```python
from build123d import *

# Parameters (mm, degrees)
F1_DEPTH  = 9.525
F6_DEPTH  = 9.525
F2_R      = 4.7625
F8_DEPTH  = 80.01
F9_W      = 12.7
F9_H      = 19.05
F10_DEPTH = 63.5
F0_W      = 12.7
F0_H      = 12.7
F11_DEPTH = 25.4
F13_DEPTH = 12.7
F14_DEPTH = 9.525


with BuildPart() as f1:
    # F0 (on Top) → F1 (new body, symmetric)
    with BuildSketch(Plane.XY):
        Polygon((-63.5, -44.45), (0, -44.45), (0, -31.75), (-50.8, -31.75), (-50.8, -6.35), (-50.8, 6.35), (-50.8, 31.75), (0, 31.75), (0, 44.45), (-63.5, 44.45), align=None)
    extrude(amount=F1_DEPTH, both=True)

    # F5 (on line) → F6 (cut, symmetric)
    with BuildSketch(Plane(origin=(-20.6375, 0, -20.6375), x_dir=(0, 1, 0), z_dir=(0.7071067812, 0, 0.7071067812))):
        Polygon((-42.8625, 39.9065859181), (-38.1, 37.156955261), (-33.3375, 39.9065859181), (-33.3375, 45.4058472321), (-38.1, 48.1554778891), (-42.8625, 45.4058472321), align=None)
        Polygon((33.3375, 39.9065859181), (38.1, 37.156955261), (42.8625, 39.9065859181), (42.8625, 45.4058472321), (38.1, 48.1554778891), (33.3375, 45.4058472321), align=None)
    extrude(amount=F6_DEPTH, both=True, mode=Mode.SUBTRACT)

    # F7: F1 across plane


with BuildPart() as f1_1:
    add(f1.part)
    add(f1.part.mirror(Plane.YZ))

    # F2 (on Front) → F8 (cut, symmetric)
    with BuildSketch(Plane.XZ):
        Circle(F2_R)
        Polygon((-10.4086411192, -0.79375), (-8.1172822383, 3.175), (-10.4086411192, 7.14375), (-14.9913588808, 7.14375), (-17.2827177617, 3.175), (-14.9913588808, -0.79375), align=None)
    extrude(amount=F8_DEPTH, both=True, mode=Mode.SUBTRACT)

    # F9 (on face) → F10 (join)
    with BuildSketch(Plane.XZ.offset(-31.75)):
        with Locations((-13.97, 0)):
            Rectangle(F9_W, F9_H)
        Polygon((-14.9913588808, -0.79375), (-17.2827177617, 3.175), (-14.9913588808, 7.14375), (-10.4086411192, 7.14375), (-8.1172822383, 3.175), (-10.4086411192, -0.79375), align=None, mode=Mode.SUBTRACT)
        Polygon((-14.9913588808, 7.14375), (-17.2827177617, 3.175), (-14.9913588808, -0.79375), (-10.4086411192, -0.79375), (-8.1172822383, 3.175), (-10.4086411192, 7.14375), align=None)
    extrude(amount=F10_DEPTH)

    # F0 (on Top) → F11 (join)
    with BuildSketch(Plane.XY):
        with Locations((-44.45, 0)):
            Rectangle(F0_W, F0_H)
    extrude(amount=F11_DEPTH)

    # F12 (on face) → F13 (join)
    with BuildSketch(Plane(origin=(0, 6.35, 0), x_dir=(-1, 0, 0), z_dir=(0, 1, 0))):
        with BuildLine():
            Line((50.8, 15.875), (50.8, 9.525))
            Line((50.8, 9.525), (57.15, 9.525))
            ThreePointArc((57.15, 9.525), (52.6598719395, 11.3848719395), (50.8, 15.875))
        make_face()
        with BuildLine():
            Line((50.8, 25.4), (50.8, 15.875))
            ThreePointArc((50.8, 15.875), (53.7052722756, 21.2094494472), (59.7626302063, 21.6626302063))
            Line((59.7626302063, 21.6626302063), (63.5, 25.4))
            Line((63.5, 25.4), (50.8, 25.4))
        make_face()
    extrude(amount=-F13_DEPTH)

    # F0 (on Top) → F14 (join)
    with BuildSketch(Plane.XY):
        with Locations((-44.45, 0)):
            Rectangle(F0_W, F0_H)
    extrude(amount=-F14_DEPTH)


solid = f1_1.part
```
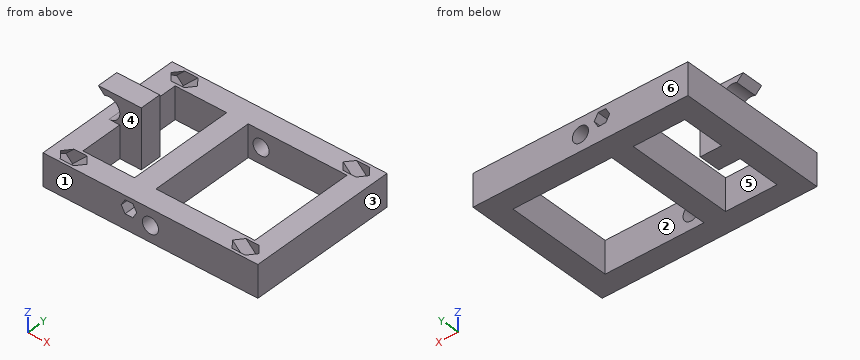
For this review, take the finished solid that the model builds, in its own axes (mm). Face numbers are marked on the shaded views. A direction names the side the tool comes from. Round coordinates to 2 decimals unless told otherwise and drop trailing zeros. Loops run counter-clockwise (first coordinate to the right, second up) from the corner with the lowest first, then second, coordinate; pieces in that order, holes last.
Q1. Add section A-A on x = 0. Give the number of separate pieces and of enclosed holes in the cut face, plus the area to 3 significant figures.
Result sheet:
separate pieces: 4
enclosed holes: 0
area: 242 mm2
Q2. Machinability: for the marked faces 4, 5 and 6, which of the approach directions +Z, -Z, +X, -X, +Y, -Y give a long, thin tool a straight path to every point of the face, cutting with its end or side? Answer none if there is none.
Result sheet:
face 4: +Z
face 5: +Z, -Z
face 6: +Z, -Z, +X, -X, +Y
Q3. Mouldability with a two-part tool opening along X and no side actions: class the marked faces 1, 2 and 3 as +X half, -X half, draft (parallel to the pull), parting line (faces both ways), or undercut.
Result sheet:
face 1: draft
face 2: undercut
face 3: +X half
Q4. Add section B-B on y = -16.5. Write out the cut boundary in (x, z) (3 decimals), plus the area to 3 significant figures.
Result sheet:
outline: (-63.5, -9.525) - (-50.8, -9.525) - (-50.8, 9.525) - (-63.5, 9.525) - close; (-20.32, -9.525) - (-7.62, -9.525) - (-7.62, 9.525) - (-20.32, 9.525) - close; (50.8, -9.525) - (63.5, -9.525) - (63.5, 9.525) - (50.8, 9.525) - close
area: 726 mm2
Q5. Add section D-D on z = 18. Write out the cut boundary in (x, y).
Result sheet:
outline: (-51.17, -6.35) - (-38.1, -6.35) - (-38.1, 6.35) - (-51.17, 6.35) - close
Q6. Add section C-C on x = 18.5. Write out the cut boundary in (y, z) (3 decimals).
Result sheet:
outline: (-44.45, -9.525) - (-31.75, -9.525) - (-31.75, 9.525) - (-44.45, 9.525) - close; (31.75, -9.525) - (44.45, -9.525) - (44.45, 9.525) - (31.75, 9.525) - close
Q7. Insertion check: pin 1 Ø3.5 at (x, y) = (-12.5, -41) entering from +Z (3 decimals); pin 2 Ø10 at (y, z) = (-6.5, 16.5) entering from -X. Each pin has a flat end and moves straight along its axis. Give the tip position at first contact, or say it passes through.
Result sheet:
pin 1: stops at z = 9.525
pin 2: stops at x = -54.2
Q8. To check wall thickness, follow line 1 along X through (y, z) = (-8, 6); line 2 along Z through (x, y) = (0, -38.5) (1 decimal); line 3 along Y through (x, z) = (39, 4). State the ranges of each line that lie inside material, in increasing order.
Result sheet:
line 1: x = -63.5 to -50.8, -20.32 to -7.62, 50.8 to 63.5
line 2: z = -9.5 to -4.8, 4.8 to 9.5
line 3: y = -44.45 to -31.75, 31.75 to 44.45
